from build123d import *

# Parameters (mm, degrees)
PAD_DEPTH     = 7.4
FILLET_R      = 5
SKETCH001_R   = 1.6
SKETCH001_R_2 = 5.1
POCKET_DEPTH  = 7.401


with BuildPart() as part:
    # Sketch → Pad (new body)
    with BuildSketch(Plane.XY):
        Polygon((90, 417.320508), (100, 400), (-30, 324.944465), (-30, 20), (0, 20), (0, 0), (-50, 0), (-50, 336.49147), align=None)
    extrude(amount=PAD_DEPTH)

    # Fillet
    fillet_edges = [part.edges().sort_by_distance(p)[0] for p in [
        (0, 0, 3.7),
        (0, 20, 3.7),
        (-50, 0, 3.7),
        (-30, 324.944465, 3.7),
        (100, 400, 3.7),
        (-30, 20, 3.7),
        (90, 417.320508, 3.7),
        (-50, 336.49147, 3.7),
    ]]
    fillet(fillet_edges, radius=FILLET_R)

    # Sketch001 (on Face5 of Fillet) → Pocket (cut, through all)
    with BuildSketch(Plane.XY.offset(7.4)):
        with Locations((86.1294, 403.538811)):
            Circle(SKETCH001_R)
        with Locations((-40, 312.17984)):
            Circle(SKETCH001_R)
        with Locations((-8.399299, 10)):
            Circle(SKETCH001_R_2)
    extrude(amount=-POCKET_DEPTH, mode=Mode.SUBTRACT)


solid = part.part
Check sheet for the modelled part. Datum: model origin and axes. Units: mm. A direction names the side the tool comes from. Round coordinates to 2 decimals unless told otherwise and drop trailing zeros. Write each loop counter-clockwise with the first axis right and the second up, starting at its lowest first coordinate (ties: lowest second). Pieces come first, ordered by that corner, then holes. Notation, with made-up numbers: (10, 8.5) -> (16, 8.5) arc R17 cw to (16, 28.5) -> close; hole circle Ø3 at (-3, 82). An arc over 180 degrees is marked (long way). Answer as CSV lines item,"result". Start each with the question number.
1) Section check A-A on y = 10. Enter the section's corners in (x, z).
2) Release check for a two-part mould opening along Y. For faces 1 (the flat face through (-30, 176, 4)), 2 (the flat face through (18.15, 375.84, 3.65)), 3 (the cylindrical face through (98.013, 400.589, 3.752)) record: pulls with the +Y half, pulls with the -Y half, needs draft (parallel to the pull), parting line crosses it, or undercut.
3) Section check D-D on x = 55. Enter the section's corners in (y, z).
4) Material ranges on line 1 (Y direction, x = -12.5, z = 4.5); line 2 (X direction, y = 37, z = 1.5); line 3 (Y direction, x = 85.5, z = 1.75), recorded low to high. Write a range as from..to.
5) Go/stop test with flat-tipped pins: P1, Ø4, axis at y = 225, z = 4.5, coming from the +X side; P2, Ø2, axis at y = 11, z = 5, coming from the +X side; P3, Ø3, axis at x = 68.5, z = 6, coming from the +Y side. Record where each tip stops, or that it passes through.
6) Section check B-B on z = 1.5. Enter the section's corners in (x, y), and give its area (3 significant figures).
7) Tool access check on faces 4 (the cylindrical face through (-3.535, 11.532, 3.752)), 5 (the flat face through (34.947, 362.442, 3.648)), 6 (the flat face through (0, 10, 4)). Record the directions out of +Z, -Z, +X, -X, +Y, -Y that give a thin tool (end or side, any length) a straight path to the whole face; none if there is none.
8) Section check C-C on y = 137. Enter the section's corners in (x, z).
Found:
1,outline,"(-50, 0) -> (-13.5, 0) -> (-13.5, 7.4) -> (-50, 7.4) -> close; (-3.3, 0) -> (0, 0) -> (0, 7.4) -> (-3.3, 7.4) -> close"
2,face 1,"undercut"
2,face 2,"pulls with the +Y half"
2,face 3,"parting line crosses it"
3,outline,"(374.02, 0) -> (397.11, 0) -> (397.11, 7.4) -> (374.02, 7.4) -> close"
4,line 1,"y = 0..6.97, 13.03..20, 335.05..358.14"
4,line 2,"x = -50..-30"
4,line 3,"y = 391.63..402.07, 405.01..414.72"
5,P1,"stops at x = -30"
5,P2,"stops at x = 0"
5,P3,"stops at y = 405.77"
6,outline,"(-50, 5) arc R5 ccw to (-45, 0) -> (-5, 0) arc R5 ccw to (0, 5) -> (0, 15) arc R5 ccw to (-5, 20) -> (-25, 20) arc R5 cw to (-30, 25) -> (-30, 322.06) arc R5 cw to (-27.5, 326.39) -> (95.67, 397.5) arc R5 ccw to (97.5, 404.33) -> (92.5, 412.99) arc R5 ccw to (85.67, 414.82) -> (-47.5, 337.93) arc R5 ccw to (-50, 333.6) -> close; hole circle Ø3.2 at (-40, 312.18); hole circle Ø10.2 at (-8.4, 10); hole circle Ø3.2 at (86.13, 403.54)"
6,area,"10,200 mm^2"
7,face 4,"+Z, -Z"
7,face 5,"+Z, -Z, +X"
7,face 6,"+Z, -Z, +X, -Y"
8,outline,"(-50, 0) -> (-30, 0) -> (-30, 7.4) -> (-50, 7.4) -> close"
